Geometry check sheet. Reference: the model listing, model coordinates, mm. A direction names the side the tool comes from. Round coordinates to 2 decimals unless told otherwise and drop trailing zeros. Order: outer loops, then holes, each group sorted by start corner. A loop starts at its lowest first (then second) coordinate and runs counter-clockwise, first axis right, second up. Notation, with made-up numbers: (59, 45) -> (79, 45) arc R29 ccw to (79, 80) -> close; hole circle Ø7 at (-37.5, 33). An arc over 180 degrees is marked (long way). Use a Markdown table: item, result. Add a question column.
Item 1: Sectioned sample at B-B, the plane z = -2.5. Record the cut outline in (x, y), and give its area (3 significant figures).
Item 2: Gauge pin test, flat ends, axial feed: pin 1 Ø2 at (x, z) = (-14.5, 0) entering from -Y; pin 2 Ø2 at (x, z) = (-15, 0) entering from +Y; pin 3 Ø6 at (x, y) = (2.5, 9) entering from -Z. Record the tip position at first contact, or that the pin passes through.
Item 3: Material ranges on probe 1 along Y at (x, z) = (5, -0.5); probe 2 along X at (y, z) = (-10.45, 0); probe 3 along X at (y, z) = (6.5, -0.5), recorded low to high. Write a range as [from, to].
Item 4: Set-up check for faces 1 (the flat face through (0, 0, -2)), 2 (the cylindrical face through (-8.17, -12.35, 0.96)), 3 (the cylindrical face through (-13.75, 12.46, -0.05)): record each of +Z, -Z, +X, -X, +Y, -Y from which the full face is reachable in a straight line by a thin tool's end or side.
Item 5: Sectioned sample at A-A, the plane x = -8.15. Record the cut outline in (y, z), and give its area (3 significant figures).
Item 6: Sectioned sample at C-C, the plane y = 13.25. Record the cut outline in (x, z), and give its area (3 significant figures).
Item 7: Mould release check, pull along X, two halves, no side actions. Record for faces 4 (the cylindrical face through (16.25, 12.46, -0.05)), 5 (the flat face through (0, -15, 1)): pulls with the +X half, pulls with the -X half, needs draft (parallel to the pull), parting line crosses it, or undercut.
Item 8: Sectioned sample at D-D, the plane y = -7.25. Record the cut outline in (x, z), and give its area (3 significant figures).
from build123d import *

# Parameters (mm, degrees)
SKETCH1_W                   = 38
SKETCH1_H                   = 30
BOSS_EXTRUDE1_DEPTH         = 4
CUT_EXTRUDE1_DEPTH          = 2
CUT_EXTRUDE2_DEPTH          = 25.939927827
TAP_DRILL_FOR_M3_TAP1_D     = 2.5
TAP_DRILL_FOR_M3_TAP1_DEPTH = 5
TAP_DRILL_FOR_M3_TAP1_TIP   = 0.751075774


with BuildPart() as part:
    # Sketch1 → Boss-Extrude1 (new, symmetric)
    with BuildSketch(Plane.XY):
        Rectangle(SKETCH1_W, SKETCH1_H)
    extrude(amount=BOSS_EXTRUDE1_DEPTH, both=True)

    # Sketch2 → Cut-Extrude1 (cut)
    with BuildSketch(Plane.XY.offset(-4)):
        with BuildLine():
            Line((-17.35, -13.2), (-17.35, -3.15))
            Line((-17.35, -3.15), (-17.35, -1.5))
            Line((-17.35, -1.5), (-17.35, 15.5))
            ThreePointArc((-17.35, 15.5), (-16.910660172, 16.560660172), (-15.85, 17))
            Line((-15.85, 17), (15.85, 17))
            ThreePointArc((15.85, 17), (16.910660172, 16.560660172), (17.35, 15.5))
            Line((17.35, 15.5), (17.35, -1.5))
            Line((17.35, -1.5), (17.35, -3.15))
            Line((17.35, -3.15), (17.35, -13.2))
            Line((17.35, -13.2), (17.35, -15))
            Line((17.35, -15), (-17.35, -15))
            Line((-17.35, -15), (-17.35, -13.2))
        make_face()
    extrude(amount=CUT_EXTRUDE1_DEPTH, mode=Mode.SUBTRACT)

    # Sketch3 → Cut-Extrude2 (cut, through all)
    with BuildSketch(Plane(origin=(0, 0, -2), x_dir=(-1, 0, 0), z_dir=(0, 0, -1))):
        with BuildLine():
            Line((9.15, 9.25), (9.15, 4.75))
            ThreePointArc((9.15, 4.75), (8.15, 3.75), (7.15, 4.75))
            Line((7.15, 4.75), (-7.15, 4.75))
            ThreePointArc((-7.15, 4.75), (-8.15, 3.75), (-9.15, 4.75))
            Line((-9.15, 4.75), (-9.15, 9.25))
            ThreePointArc((-9.15, 9.25), (-8.15, 10.25), (-7.15, 9.25))
            Line((-7.15, 9.25), (7.15, 9.25))
            ThreePointArc((7.15, 9.25), (8.15, 10.25), (9.15, 9.25))
        make_face()
        with BuildLine():
            Line((-7.15, -6.85), (7.15, -6.85))
            ThreePointArc((7.15, -6.85), (8.15, -5.85), (9.15, -6.85))
            Line((9.15, -6.85), (9.15, -11.35))
            ThreePointArc((9.15, -11.35), (8.15, -12.35), (7.15, -11.35))
            Line((7.15, -11.35), (-7.15, -11.35))
            ThreePointArc((-7.15, -11.35), (-8.15, -12.35), (-9.15, -11.35))
            Line((-9.15, -11.35), (-9.15, -6.85))
            ThreePointArc((-9.15, -6.85), (-8.15, -5.85), (-7.15, -6.85))
        make_face()
    extrude(amount=-CUT_EXTRUDE2_DEPTH, mode=Mode.SUBTRACT)

    # Sketch5 → M3 Tapped Hole1 (revolve, cut)
    with BuildSketch(Plane(origin=(14.5, -15, 0), x_dir=(0, 0, -1), z_dir=(1, 0, 0))):
        Polygon((0, 0), (0, 6.751075774), (1.25, 6), (1.25, 0), align=None)
    m3_tapped_hole1 = revolve(axis=Axis((14.5, -21.35, 0), (0, 1, 0)), mode=Mode.SUBTRACT)

    # Mirror1: M3 Tapped Hole1 across plane
    add(m3_tapped_hole1.mirror(Plane(origin=(0, 0, 0), x_dir=(0, 0, 1), z_dir=(1, 0, 0))), mode=Mode.SUBTRACT)

    # Tap Drill for M3 Tap1
    with Locations(Plane(origin=(0, 15, 0), x_dir=(1, 0, 0), z_dir=(0, 1, 0))):
        with Locations((15, 0), (-15, 0)):
            Hole(TAP_DRILL_FOR_M3_TAP1_D / 2, depth=TAP_DRILL_FOR_M3_TAP1_DEPTH)
            with Locations((0, 0, -(TAP_DRILL_FOR_M3_TAP1_DEPTH + TAP_DRILL_FOR_M3_TAP1_TIP / 2))):  # 118° drill point
                Cone(0, TAP_DRILL_FOR_M3_TAP1_D / 2, TAP_DRILL_FOR_M3_TAP1_TIP, mode=Mode.SUBTRACT)


solid = part.part
Found:
| question | item | result |
|---|---|---|
| 1 | outline | (-19, -15) -> (-17.35, -15) -> (-17.35, 15) -> (-19, 15) -> close; (17.35, -15) -> (19, -15) -> (19, 15) -> (17.35, 15) -> close |
| 1 | area | 99.0 mm2 |
| 2 | pin 1 | stops at y = -8.85 |
| 2 | pin 2 | stops at y = 9.85 |
| 2 | pin 3 | stops at z = -2 |
| 3 | probe 1 | y = [-15, -11.35], [-6.85, 4.75], [9.25, 15] |
| 3 | probe 2 | x = [-19, -15.75], [-13.25, -9.15], [9.15, 13.25], [15.75, 19] |
| 3 | probe 3 | x = [-19, -9.15], [9.15, 19] |
| 4 | face 1 | -Z, +Y, -Y |
| 4 | face 2 | +Z, -Z |
| 4 | face 3 | +Y |
| 5 | outline | (-15, -2) -> (-12.35, -2) -> (-12.35, 4) -> (-15, 4) -> close; (-5.85, -2) -> (3.75, -2) -> (3.75, 4) -> (-5.85, 4) -> close; (10.25, -2) -> (15, -2) -> (15, 4) -> (10.25, 4) -> close |
| 5 | area | 102 mm2 |
| 6 | outline | (-19, -4) -> (-17.35, -4) -> (-17.35, -2) -> (17.35, -2) -> (17.35, -4) -> (19, -4) -> (19, 4) -> (-19, 4) -> close; hole circle Ø2.5 at (-15, 0); hole circle Ø2.5 at (15, 0) |
| 6 | area | 225 mm2 |
| 7 | face 4 | undercut |
| 7 | face 5 | needs draft |
| 8 | outline | (-19, -4) -> (-17.35, -4) -> (-17.35, -2) -> (-9.15, -2) -> (-9.15, 4) -> (-19, 4) -> close; (9.15, -2) -> (17.35, -2) -> (17.35, -4) -> (19, -4) -> (19, 4) -> (9.15, 4) -> close |
| 8 | area | 125 mm2 |
